Verification items for this drawing (mm, ordinates from the low corner). A direction names the side the tool comes from. Give positions to 0.01 mm unless a question says otherwise; leave off trailing zeros. Write each loop counter-clockwise with the first axis right and the second up, starting at its lowest first coordinate (ties: lowest second). Pieces come first, ordered by that corner, then holes. Notation, with made-up numbers: (75, -12.75) -> (113, -12.75) arc R21 cw to (113, 24.25) -> close; hole circle Ø3 at (-27.5, 87). An arc over 180 degrees is marked (long way). One line per item, written item: value.
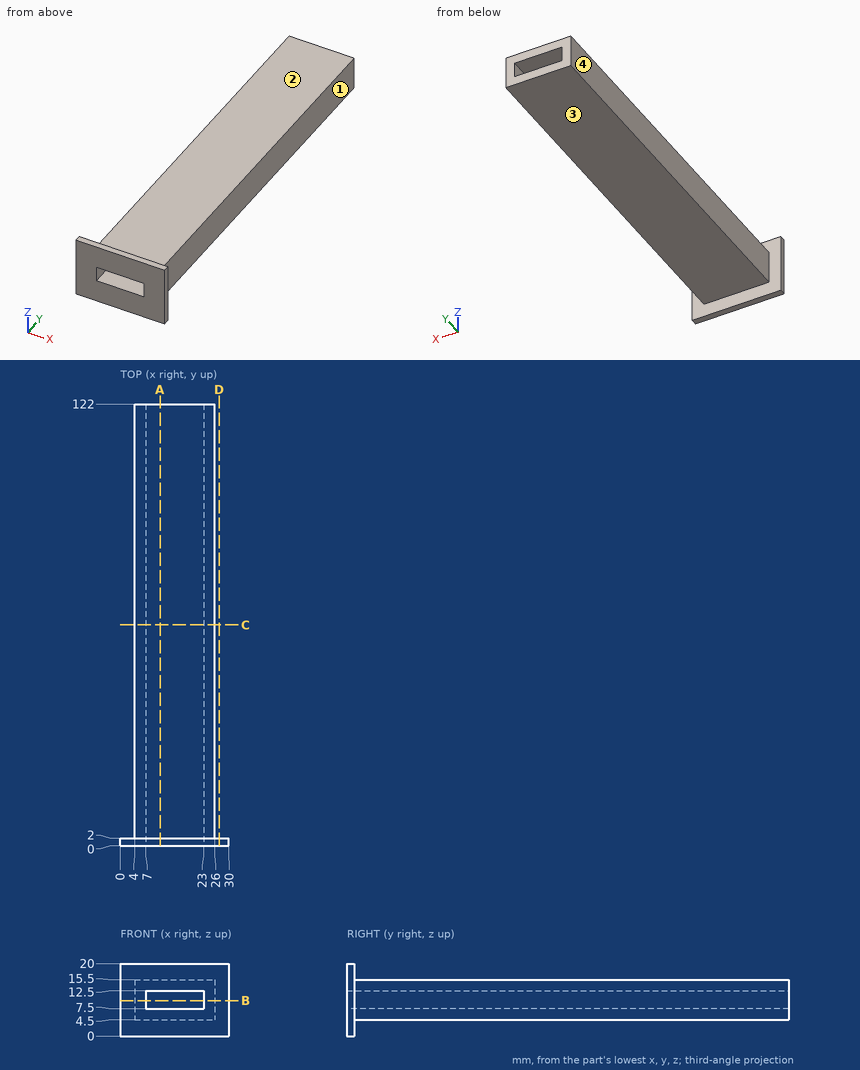
1) Sectioned sample at B-B on z = 9.75. Record the cut outline in (x, y), plus the area to 3 significant figures.
Verdict:
outline: (0, 0) -> (7, 0) -> (7, 122) -> (4, 122) -> (4, 2) -> (0, 2) -> close; (23, 0) -> (30, 0) -> (30, 2) -> (26, 2) -> (26, 122) -> (23, 122) -> close
area: 748 mm^2
2) Sectioned sample at C-C on y = 61. Record the cut outline in (x, z), plus the area to 3 significant figures.
Verdict:
outline: (4, 4.5) -> (26, 4.5) -> (26, 15.5) -> (4, 15.5) -> close; hole (7, 7.5) -> (23, 7.5) -> (23, 12.5) -> (7, 12.5) -> close
area: 162 mm^2
3) Depth check by flat-ended pin: pin 1 Ø5 at (x, y) = (7, 50.5) entering from -Z; pin 2 Ø17.5 at (x, y) = (15, 58) entering from +Z; pin 3 Ø1.5 at (y, z) = (81.5, 10.5) entering from -X; pin 4 Ø10 at (x, z) = (17, 8) entering from +Y. Enter the tip coordinate at first touch or a pass-through.
Verdict:
pin 1: z = 4.5
pin 2: z = 15.5
pin 3: x = 4
pin 4: y = 122
4) Sectioned sample at A-A on x = 11. Record the cut outline in (y, z), plus the area to 3 significant figures.
Verdict:
outline: (0, 0) -> (2, 0) -> (2, 4.5) -> (122, 4.5) -> (122, 7.5) -> (0, 7.5) -> close; (0, 12.5) -> (122, 12.5) -> (122, 15.5) -> (2, 15.5) -> (2, 20) -> (0, 20) -> close
area: 750 mm^2
5) Scan lines: probe 1 along Z at (x, y) = (11.25, 9); probe 2 along X at (y, z) = (95, 8); probe 3 along X at (y, z) = (111, 5.75). Record each from-to range of solid material in increasing order.
Verdict:
probe 1: 4.5 to 7.5, 12.5 to 15.5
probe 2: 4 to 7, 23 to 26
probe 3: 4 to 26
6) Tool access check on the marked faces 1, 2, 3 and 4. Record the directions out of +Z, -Z, +X, -X, +Y, -Y that give a thin tool (end or side, any length) a straight path to the whole face; none if there is none.
Verdict:
face 1: +Z, -Z, +X, +Y
face 2: +Z, +X, -X, +Y
face 3: -Z, +X, -X, +Y
face 4: +Z, -Z, -X, +Y
7) Sectioned sample at D-D on x = 27.25. Record the cut outline in (y, z).
Verdict:
outline: (0, 0) -> (2, 0) -> (2, 20) -> (0, 20) -> close
